from build123d import *

# Parameters (mm, degrees)
F1_DEPTH = 25.4
F2_DEPTH = 25.4
F4_DEPTH = 25.4
F5_DEPTH = 25.4


with BuildPart() as f1:
    # F0 (on Front) → F1 (new body)
    with BuildSketch(Plane.XZ):
        Polygon((-21.2792549282, 28.9397872984), (-33.6739535907, 26.1718557484), (-33.6739535907, -5.5781442516), (4.4260464093, -5.5781442516), (4.4260464093, 7.1218557484), (-8.2739535907, 7.1218557484), align=None)
    extrude(amount=F1_DEPTH)

    # F2 (add): a face of the model
    f2_faces = [f1.faces().sort_by_distance(p)[0] for p in [
        (-18.6613811505, -25.4, 7.7485425126),
    ]]
    extrude(f2_faces, amount=F2_DEPTH)

    # F3 (on Front) → F4 (join)
    with BuildSketch(Plane.XZ):
        Polygon((-33.7073244154, 26.1170342565), (-21.333374083, 28.9452429861), (-33.7073244154, 28.9452429861), align=None)
    extrude(amount=F4_DEPTH)

    # F5 (cut): a face of the model
    f5_faces = [f1.faces().sort_by_distance(p)[0] for p in [
        (-18.6613811505, -50.8, 7.7485425126),
    ]]
    extrude(f5_faces, amount=-F5_DEPTH, mode=Mode.SUBTRACT)


solid = f1.part
Work out the finished part from the listing and answer in its coordinate system (mm). Round coordinates to 2 decimals unless told otherwise and drop trailing zeros. Write each loop counter-clockwise with the first axis right and the second up, starting at its lowest first coordinate (ties: lowest second). Pieces come first, ordered by that corner, then holes. Notation, with made-up numbers: (70, -34) -> (76, -34) arc R11 ccw to (76, -19) -> close; hole circle Ø4 at (-3, -15). An arc over 180 degrees is marked (long way). Answer as CSV lines item,"result". Start each with the question number.
(1) Each of these flat-tipped pins is pushed along its axis until it touches: pin 1 (2 mm diameter, centred on x = -17, z = 15, fed in from +Y); pin 2 (12 mm diameter, centred on x = -3, z = 21, fed in from -Y); pin 3 (4 mm diameter, centred on y = -4, z = 15.5, fed in from +X); pin 4 (10 mm diameter, centred on x = -15, y = -18.5, fed in from +Z). Where does it stop, or does it pass through?
(2) Find the intervals of material crossed by probe 1 along X at (y, z) = (-1.75, -1); probe 2 along Z at (x, y) = (-2.5, -14.5); probe 3 along X at (y, z) = (-4.5, 24), in increasing order.
(3) The part is cut by section C-C, the plane z = 21. Give the vertices of the cut face in (x, y).
(4) The part is cut by section B-B, the plane x = -6. Give the vertices of the cut face in (y, z).
Output values:
1,pin 1,"stops at y = 0"
1,pin 2,"passes through"
1,pin 3,"stops at x = -12.08"
1,pin 4,"stops at z = 26.79"
2,probe 1,"x = -33.67 to 4.43"
2,probe 2,"z = -5.58 to 7.12"
2,probe 3,"x = -33.67 to -18.33"
3,outline,"(-33.67, -25.4) -> (-16.55, -25.4) -> (-16.55, 0) -> (-33.67, 0) -> close"
4,outline,"(-25.4, -5.58) -> (0, -5.58) -> (0, 7.12) -> (-25.4, 7.12) -> close"
